from build123d import *

# Parameters (mm, degrees)
F0_R     = 100
F1_DEPTH = 60
F2_R     = 97
F2_R_2   = 5
F3_DEPTH = 57


with BuildPart() as f1:
    # F0 (on Top) → F1 (new body)
    with BuildSketch(Plane.XY):
        Circle(F0_R)
        with BuildLine():
            ThreePointArc((-55.621778, -35), (-65.451407, -36.294095), (-56.291651, -32.5))
            ThreePointArc((-56.291651, -32.5), (-55.792149, -33.705905), (-55.621778, -35))
        make_face(mode=Mode.SUBTRACT)
        with BuildLine():
            ThreePointArc((5, -70), (-3.535534, -73.535534), (0, -65))
            ThreePointArc((0, -65), (3.535534, -66.464466), (5, -70))
        make_face(mode=Mode.SUBTRACT)
        with BuildLine():
            ThreePointArc((65.621778, -35), (59.327683, -39.829629), (56.291651, -32.5))
            ThreePointArc((56.291651, -32.5), (61.915873, -30.170371), (65.621778, -35))
        make_face(mode=Mode.SUBTRACT)
        with BuildLine():
            ThreePointArc((-55.621778, 35), (-55.792149, 33.705905), (-56.291651, 32.5))
            ThreePointArc((-56.291651, 32.5), (-65.451407, 36.294095), (-55.621778, 35))
        make_face(mode=Mode.SUBTRACT)
        with BuildLine():
            ThreePointArc((65.621778, 35), (61.915873, 30.170371), (56.291651, 32.5))
            ThreePointArc((56.291651, 32.5), (59.327683, 39.829629), (65.621778, 35))
        make_face(mode=Mode.SUBTRACT)
        with BuildLine():
            ThreePointArc((5, 70), (3.535534, 66.464466), (0, 65))
            ThreePointArc((0, 65), (-3.535534, 73.535534), (5, 70))
        make_face(mode=Mode.SUBTRACT)
    extrude(amount=F1_DEPTH)

    # F2 (on face) → F3 (cut)
    with BuildSketch(Plane.XY.offset(60)):
        Circle(F2_R)
        Circle(F2_R)
        with Locations((-60.621778, -35)):
            Circle(F2_R_2, mode=Mode.SUBTRACT)
        with Locations((0, -70)):
            Circle(F2_R_2, mode=Mode.SUBTRACT)
        with Locations((60.621778, -35)):
            Circle(F2_R_2, mode=Mode.SUBTRACT)
        with Locations((-60.621778, 35)):
            Circle(F2_R_2, mode=Mode.SUBTRACT)
        with Locations((60.621778, 35)):
            Circle(F2_R_2, mode=Mode.SUBTRACT)
        with Locations((0, 70)):
            Circle(F2_R_2, mode=Mode.SUBTRACT)
    extrude(amount=-F3_DEPTH, mode=Mode.SUBTRACT)


solid = f1.part
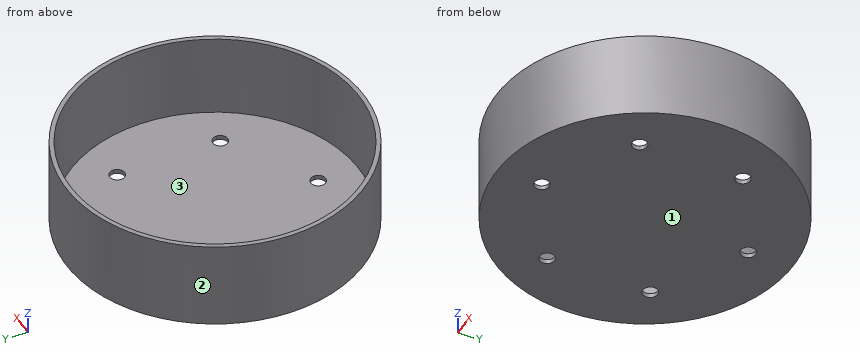
Geometry check sheet. Reference: the model listing, model coordinates, mm. Face numbers are marked on the shaded views. Give positions to 0.01 mm unless a question says otherwise; leave off trailing zeros. Order: outer loops, then holes, each group sorted by start corner. A loop starts at its lowest first (then second) coordinate and runs counter-clockwise, first axis right, second up.
1) Cross-section at A-A (y = 0). Record the boundary of the cut face in (x, z), then the cut area to 3 significant figures.
Results are:
outline: (-100, 0) - (100, 0) - (100, 60) - (97, 60) - (97, 3) - (-97, 3) - (-97, 60) - (-100, 60) - close
area: 942 mm2
2) Material ranges on probe 1 along Y at (x, z) = (0, 1.25); probe 2 along X at (y, z) = (-2.5, 56.5); probe 3 along Y at (x, z) = (0, 29), recorded low to high.
Results are:
probe 1: y = -100 to -75, -65 to 65, 75 to 100
probe 2: x = -99.97 to -96.97, 96.97 to 99.97
probe 3: y = -100 to -97, 97 to 100
3) Draft check along Y on the marked faces 1, 2 and 3. Enter one of: released by +Y, released by -Y, zero draft, split by the parting line, or undercut.
Results are:
face 1: zero draft
face 2: split by the parting line
face 3: undercut
4) Cross-section at B-B (x = 52.5). Record the boundary of the cut face in (y, z).
Results are:
outline: (-85.11, 0) - (85.11, 0) - (85.11, 60) - (81.56, 60) - (81.56, 3) - (-81.56, 3) - (-81.56, 60) - (-85.11, 60) - close
5) Cross-section at C-C (z = 23.5). Record the boundary of the cut face in (x, y).
Results are:
outline: circle Ø200 at (0, 0); hole circle Ø194 at (0, 0)
6) Gauge pin test, flat ends, axial feed: pin 1 (2 mm diameter, centred on x = -15, y = -3.5, fed in from +Z); pin 2 (8 mm diameter, centred on x = 78.5, z = 39, fed in from +Y); pin 3 (1.5 mm diameter, centred on y = 56.5, z = 47, fed in from +X). Record the tip position at first contact, or that the pin passes through.
Results are:
pin 1: stops at z = 3
pin 2: stops at y = 66.71
pin 3: stops at x = 83.02
